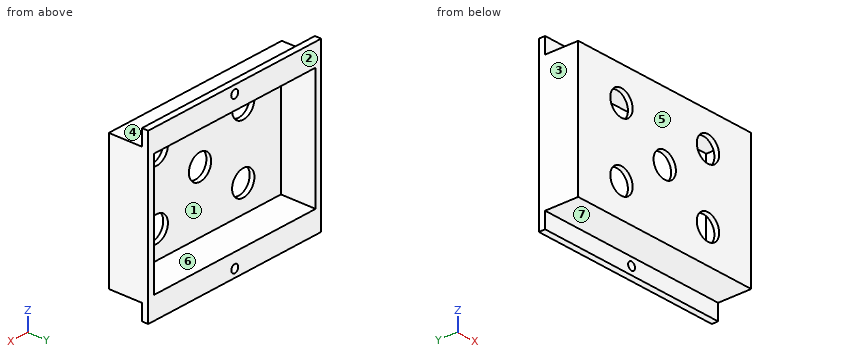
```python
from build123d import *

# Parameters (mm, degrees)
SKETCH1_W           = 124
SKETCH1_H           = 84
BOSS_EXTRUDE1_DEPTH = 25
SKETCH2_W           = 116
SKETCH2_H           = 76
CUT_EXTRUDE1_DEPTH  = 22
SKETCH3_R           = 8
CUT_EXTRUDE2_DEPTH  = 79.051265204
SKETCH4_W           = 124
SKETCH4_H           = 4
BOSS_EXTRUDE2_DEPTH = 10
SKETCH5_W           = 124
SKETCH5_H           = 4
BOSS_EXTRUDE3_DEPTH = 10
SKETCH6_R           = 2.5
CUT_EXTRUDE3_DEPTH  = 85.693565281


with BuildPart() as part:
    # Sketch1 → Boss-Extrude1 (new body)
    with BuildSketch(Plane(origin=(0, 0, 0), x_dir=(1, 0, 0), z_dir=(0, 1, 0))):
        Rectangle(SKETCH1_W, SKETCH1_H)
    extrude(amount=BOSS_EXTRUDE1_DEPTH)

    # Sketch2 → Cut-Extrude1 (cut)
    with BuildSketch(Plane(origin=(0, 25, 0), x_dir=(1, 0, 0), z_dir=(0, 1, 0))):
        Rectangle(SKETCH2_W, SKETCH2_H)
    extrude(amount=-CUT_EXTRUDE1_DEPTH, mode=Mode.SUBTRACT)

    # Sketch3 → Cut-Extrude2 (cut, through all)
    with BuildSketch(Plane(origin=(0, 3, 0), x_dir=(1, 0, 0), z_dir=(0, 1, 0))):
        with Locations(Location((0, 0, 0), (0, 0, 270))):
            Circle(SKETCH3_R)
        with Locations(Location((-31, 21, 0), (0, 0, 270))):
            Circle(SKETCH3_R)
        with Locations(Location((-31, -21, 0), (0, 0, 270))):
            Circle(SKETCH3_R)
        with Locations(Location((31, 21, 0), (0, 0, 270))):
            Circle(SKETCH3_R)
        with Locations(Location((31, -21, 0), (0, 0, 270))):
            Circle(SKETCH3_R)
    extrude(amount=-CUT_EXTRUDE2_DEPTH, mode=Mode.SUBTRACT)

    # Sketch4 → Boss-Extrude2 (add)
    with BuildSketch(Plane.XY.offset(42)):
        with Locations((0, 23)):
            Rectangle(SKETCH4_W, SKETCH4_H)
    extrude(amount=BOSS_EXTRUDE2_DEPTH)

    # Sketch5 → Boss-Extrude3 (add)
    with BuildSketch(Plane(origin=(0, 0, -42), x_dir=(-1, 0, 0), z_dir=(0, 0, -1))):
        with Locations((0, 23)):
            Rectangle(SKETCH5_W, SKETCH5_H)
    extrude(amount=BOSS_EXTRUDE3_DEPTH)

    # Sketch6 → Cut-Extrude3 (cut, through all)
    with BuildSketch(Plane(origin=(0, 25, 0), x_dir=(1, 0, 0), z_dir=(0, 1, 0))):
        with Locations(Location((0, 47, 0), (0, 0, 270))):
            Circle(SKETCH6_R)
        with Locations(Location((0, -47, 0), (0, 0, 270))):
            Circle(SKETCH6_R)
    extrude(amount=-CUT_EXTRUDE3_DEPTH, mode=Mode.SUBTRACT)


solid = part.part
```
Could you check a few things on this model? Use its own coordinates, in mm. Face numbers are marked on the shaded views. A direction names the side the tool comes from. Round coordinates to 2 decimals unless told otherwise and drop trailing zeros. Order: outer loops, then holes, each group sorted by start corner. A loop starts at its lowest first (then second) coordinate and runs counter-clockwise, first axis right, second up. Notation, with made-up numbers: M 70,12.5 L 114,12.5 A16 ccw 114,20.5 Z; hole C 40.5,70 d8. An arc over 180 degrees is marked long. One line per question, with ' | ' between items. Start each with the question number.
(1) Suppose I cut it at A-A on z = -47. List the corners of the cut face in (x, y) for me.
(2) For P1, Ø10.5, axis at x = 26, y = 10, coming from the -Z side; P2, Ø8, axis at x = 10.5, z = 48.5, coming from the -Y side; P3, Ø18.5, axis at x = 0, z = 0, coming from the +Y side, each with a flat end and sliding along its axis, tell me the tip position at first contact or that it passes through.
(3) Suppose I cut it at D-D on x = 31. List the corners of the cut face in (y, z) for me, then the cut area to 3 significant figures.
(4) Thinking about a two-plate mould opening in X: for the marked faces 1, 2 and 3, which applies, +X half, -X half, draft (parallel to the pull), parting line (faces both ways), or undercut?
(5) Suppose I cut it at B-B on x = 0. List the corners of the cut face in (y, z) for me, then the cut area to 3 significant figures.
(6) Suppose I cut it at C-C on y = 23.25. List the corners of the cut face in (x, z) for me.
(7) For the marked faces 4, 5, 6 and 7, which set-ups out of +Z, -Z, +X, -X, +Y, -Y let a thin tool reach every point of the face, with its end or its side?
(8) Please list where these lines run through material, in increasing order: line 1 along X through (y, z) = (1.4, 21); line 2 along Z through (x, y) = (16, 3.5); line 3 along X through (y, z) = (17.5, 26.5).
Geometry results:
1) outline: M -62,21 L -2.5,21 L -2.5,25 L -62,25 Z; M 2.5,21 L 62,21 L 62,25 L 2.5,25 Z
2) P1: z = -42 | P2: y = 21 | P3: y = 3
3) outline: M 0,-42 L 21,-42 L 21,-52 L 25,-52 L 25,-38 L 3,-38 L 3,-29 L 0,-29 Z; M 0,-13 L 3,-13 L 3,13 L 0,13 Z; M 0,29 L 3,29 L 3,38 L 25,38 L 25,52 L 21,52 L 21,42 L 0,42 Z | area: 412 mm²
4) face 1: undercut | face 2: draft | face 3: -X half
5) outline: M 0,-42 L 21,-42 L 21,-44.5 L 25,-44.5 L 25,-38 L 3,-38 L 3,-8 L 0,-8 Z; M 0,8 L 3,8 L 3,38 L 25,38 L 25,44.5 L 21,44.5 L 21,42 L 0,42 Z; M 21,-52 L 25,-52 L 25,-49.5 L 21,-49.5 Z; M 21,49.5 L 25,49.5 L 25,52 L 21,52 Z | area: 420 mm²
6) outline: M -62,-52 L 62,-52 L 62,52 L -62,52 Z; hole M -58,-38 L 58,-38 L 58,38 L -58,38 Z; hole C 0,-47 d5; hole C 0,47 d5
7) face 4: +Z, +X, -X, -Y | face 5: +Z, -Z, +X, -X, -Y | face 6: +Y | face 7: -Z, +X, -X, -Y
8) line 1: -62 to -39, -23 to 23, 39 to 62 | line 2: -42 to -38, 38 to 42 | line 3: -62 to -58, 58 to 62
